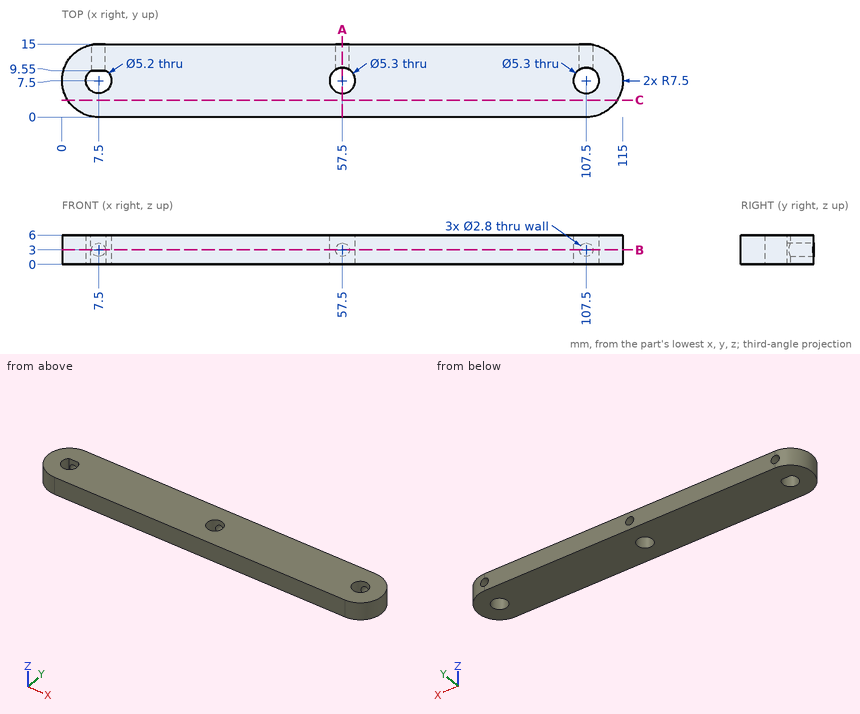
Source: three-view drawing plus pictorial views. Frame: mm from the lowest corner of the part. Give positions to 0.01 mm unless a question says otherwise; leave off trailing zeros. Write each loop counter-clockwise with the first axis right and the second up, starting at its lowest first coordinate (ties: lowest second). Pieces come first, ordered by that corner, then holes. Notation, with made-up numbers: (8.25, 83.5) -> (16.25, 83.5) arc R26 cw to (16.25, 119.5) -> close; hole circle Ø11 at (21, 51). An arc over 180 degrees is marked (long way). Answer in a Markdown table with one row per item.
(1) Section query C-C on y = 3.5. Return loops of the section in (x, z), then the cut area to 3 significant figures.
Answers below:
| item | result |
|---|---|
| outline | (1.16, 0) -> (113.84, 0) -> (113.84, 6) -> (1.16, 6) -> close |
| area | 676 mm^2 |
(2) Section query A-A on x = 57.5. Return loops of the section in (y, z).
Answers below:
| item | result |
|---|---|
| outline | (0, 0) -> (4.85, 0) -> (4.85, 6) -> (0, 6) -> close; (10.15, 0) -> (15, 0) -> (15, 1.6) -> (10.15, 1.6) -> close; (10.15, 4.4) -> (15, 4.4) -> (15, 6) -> (10.15, 6) -> close |
(3) Pin query (flat end, axial travel): pin 1 (3 mm diameter, centred on y = 11, z = 2.5, fed in from +X); pin 2 (1 mm diameter, centred on y = 11.5, z = 1, fed in from +X); pin 3 (2 mm diameter, centred on y = 13, z = 3.5, fed in from -X). Return the tip coordinate at first contact, or that it passes through.
Answers below:
| item | result |
|---|---|
| pin 1 | x = 114.73 |
| pin 2 | x = 114.13 |
| pin 3 | x = 1.5 |
(4) Ray query, line 1 along X through (y, z) = (6, 3); line 2 along X through (y, z) = (13, 3.5); line 3 along Y through (x, z) = (57, 5.5). Return the intervals inside material, ascending. Write a range as [from, to].
Answers below:
| item | result |
|---|---|
| line 1 | [0.15, 5.38], [9.62, 55.32], [59.68, 105.32], [109.68, 114.85] |
| line 2 | [2.4, 6.19], [8.81, 56.19], [58.81, 106.19], [108.81, 112.6] |
| line 3 | [0, 4.9], [10.1, 15] |
(5) Section query B-B on z = 3. Return loops of the section in (x, y).
Answers below:
| item | result |
|---|---|
| outline | (5.9, 9.55) -> (6.1, 9.55) -> (6.1, 14.87) arc R7.5 ccw to (7.5, 0) -> (107.5, 0) arc R7.5 ccw to (108.9, 14.87) -> (108.9, 9.75) arc R2.65 cw (long way) to (106.1, 9.75) -> (106.1, 15) -> (58.9, 15) -> (58.9, 9.75) arc R2.65 cw (long way) to (56.1, 9.75) -> (56.1, 15) -> (8.9, 15) -> (8.9, 9.55) -> (9.1, 9.55) arc R2.6 cw (long way) to start |
